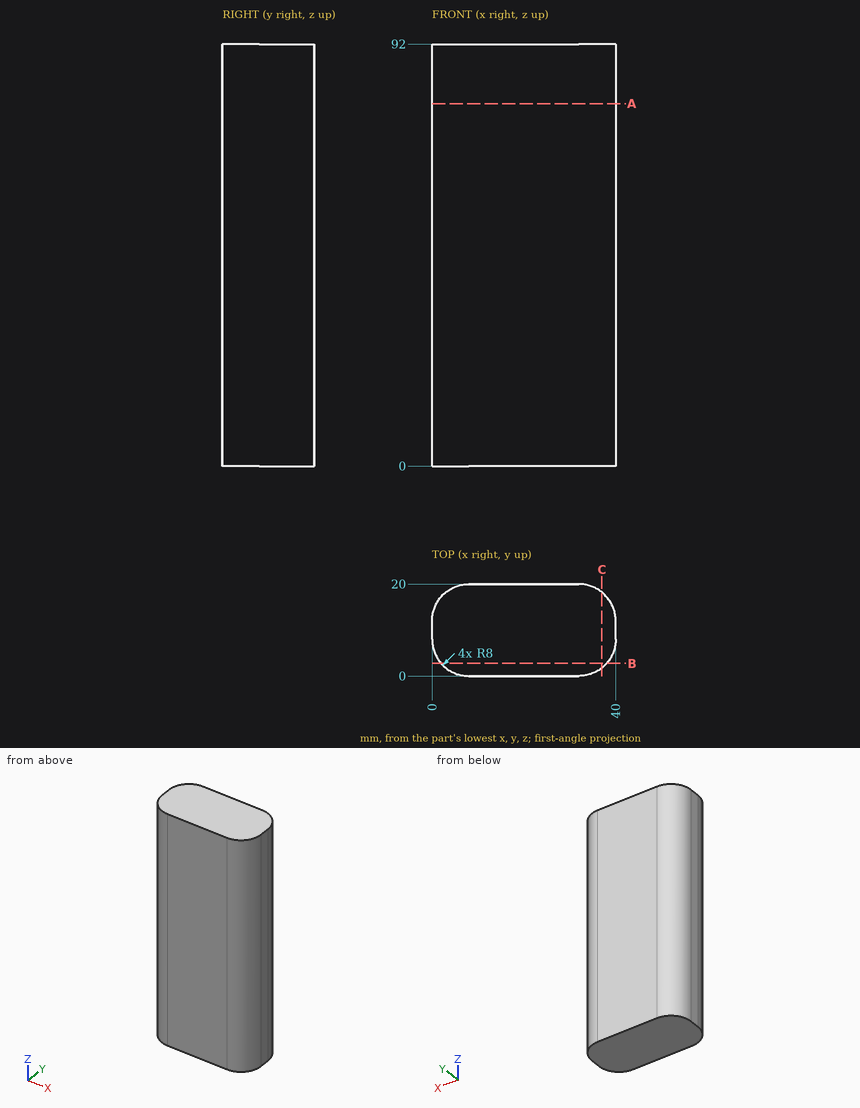
Can you work these out from the drawing? Everything is in mm from the part's minimum corner. Round coordinates to 2 decimals unless told otherwise and drop trailing zeros. Loops run counter-clockwise (first coordinate to the right, second up) from the corner with the lowest first, then second, coordinate; pieces in that order, holes last. Notation, with made-up numbers: (15.5, -15.75) -> (24.5, -15.75) arc R29 cw to (24.5, 6.25) -> close; hole circle Ø8 at (88.25, 54.5). An arc over 180 degrees is marked (long way). Put each result on its own line as item: value.
Q1. Please list where these lines run through material, in increasing order: line 1 (X direction, y = 3.75, z = 35); line 2 (X direction, y = 1.25, z = 39.5); line 3 (Y direction, x = 4.5, z = 65). Write a range as from..to.
Checks:
line 1: 1.22..38.78
line 2: 3.71..36.29
line 3: 0.81..19.19
Q2. For pin 1 Ø1 at (x, z) = (7, 24.5) entering from -Y; pin 2 Ø1 at (y, z) = (15.5, 63.5) entering from -X, each with a flat end and sliding along its axis, tell me the tip position at first contact or that it passes through.
Checks:
pin 1: y = 0.02
pin 2: x = 0.58
Q3. I want a section at B-B on y = 2.75. Write out the boundary of the cut face in (x, z).
Checks:
outline: (1.96, 0) -> (38.04, 0) -> (38.04, 92) -> (1.96, 92) -> close
Q4. I want a section at C-C on x = 37. Write out the boundary of the cut face in (y, z) (3 decimals).
Checks:
outline: (1.755, 0) -> (18.245, 0) -> (18.245, 92) -> (1.755, 92) -> close
Q5. I want a section at A-A on z = 79. Write out the boundary of the cut face in (x, y).
Checks:
outline: (0, 8) arc R8 ccw to (8, 0) -> (32, 0) arc R8 ccw to (40, 8) -> (40, 12) arc R8 ccw to (32, 20) -> (8, 20) arc R8 ccw to (0, 12) -> close
